from build123d import *

# Parameters (mm, degrees)
F0_R     = 25.4
F1_DEPTH = 25.4
F2_T     = -2.54
F3_R     = 10.031251
F4_DEPTH = 25.401


with BuildPart() as f1:
    # F0 (on Front) → F1 (new body)
    with BuildSketch(Plane.XZ):
        Circle(F0_R)
    extrude(amount=F1_DEPTH)

    # F2
    f2_openings = [f1.faces().sort_by_distance(p)[0] for p in [
        (0, 0, 0),
    ]]
    offset(amount=F2_T, openings=f2_openings)

    # F3 (on Right) → F4 (cut, through all)
    with BuildSketch(Plane.YZ):
        with Locations((-12.55889, 0)):
            Circle(F3_R)
    extrude(amount=-F4_DEPTH, mode=Mode.SUBTRACT)


solid = f1.part
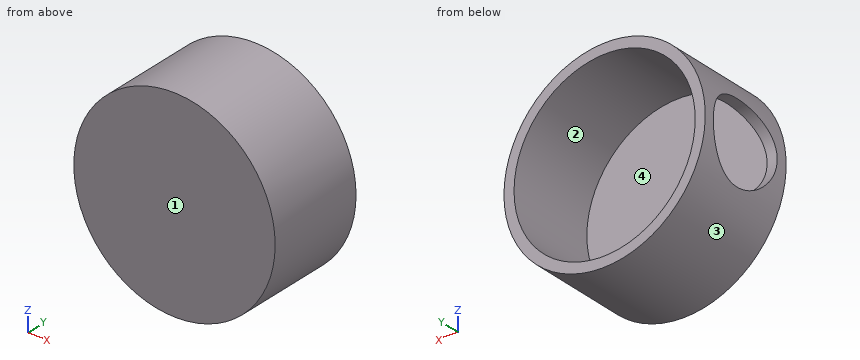
Source: CAD feature listing. Evaluate the final solid. Frame: model axes, mm. Face numbers are marked on the shaded views. Coordinates: 2 decimals unless noted, no trailing zeros. Loops run counter-clockwise (first coordinate to the right, second up) from the corner with the lowest first, then second, coordinate; pieces in that order, holes last. Notation, with made-up numbers: (23, 68.25) -> (59, 68.25) arc R13 ccw to (59, 76.25) -> close; hole circle Ø5 at (51, 62.5). An arc over 180 degrees is marked (long way). Answer in a Markdown table with one row per item. Add a question column.
Q1. Contact query for flat-ended pins moving along their axis: pin 1 Ø6 at (x, z) = (-7, 10.5) entering from +Y; pin 2 Ø10 at (x, y) = (-17.5, -4.5) entering from +Z; pin 3 Ø8 at (x, y) = (4, -20.5) entering from -Z. Output: stop coordinate, or through.
Q2. Section B-B on x = 0. Return the cut outline in (y, z), and give its area (3 significant figures).
Q3. Ray query, line 1 along Z through (x, y) = (0, -9.5); line 2 along Y through (x, z) = (1.5, 8.5); line 3 along X through (y, z) = (-7, 18). Return the intervals inside material, ascending.
Q4. Pull-direction query (X, two-part tool) for the marked faces 1, 2, 3 and 4; classes: pulls with the +X half, pulls with the -X half, needs draft (parallel to the pull), parting line crosses it, or undercut.
Q5. Section C-C on z = 19.5. Return the cut outline in (x, y), and give its area (3 significant figures).
Q6. Section A-A on z = 0. Return the cut outline in (x, y), and give its area (3 significant figures).
Q7. Section D-D on y = -15. Return the cut outline in (x, z).
Computed values:
| question | item | result |
|---|---|---|
| 1 | pin 1 | stops at y = -22.86 |
| 1 | pin 2 | stops at z = 22.11 |
| 1 | pin 3 | stops at z = -25.4 |
| 2 | outline | (-25.4, -25.4) -> (0, -25.4) -> (0, -22.86) -> (-22.86, -22.86) -> (-22.86, 22.86) -> (0, 22.86) -> (0, 25.4) -> (-25.4, 25.4) -> close |
| 2 | area | 245 mm^2 |
| 3 | line 1 | z = -25.4 to -22.86, 22.86 to 25.4 |
| 3 | line 2 | y = -25.4 to -22.86 |
| 3 | line 3 | x = -17.92 to -14.09, 14.09 to 17.92 |
| 4 | face 1 | needs draft |
| 4 | face 2 | undercut |
| 4 | face 3 | parting line crosses it |
| 4 | face 4 | undercut |
| 5 | outline | (-16.28, -25.4) -> (16.28, -25.4) -> (16.28, 0) -> (11.93, 0) -> (11.93, -22.86) -> (-11.93, -22.86) -> (-11.93, 0) -> (-16.28, 0) -> close |
| 5 | area | 281 mm^2 |
| 6 | outline | (-25.4, -25.4) -> (25.4, -25.4) -> (25.4, 0) -> (22.86, 0) -> (22.86, -22.86) -> (-22.86, -22.86) -> (-22.86, -22.59) -> (-25.4, -22.59) -> close; (-25.4, -2.53) -> (-22.86, -2.53) -> (-22.86, 0) -> (-25.4, 0) -> close |
| 6 | area | 194 mm^2 |
| 7 | outline | (-23.46, -9.73) arc R25.4 ccw (long way) to (-23.46, 9.73) -> (-20.69, 9.73) arc R22.86 cw (long way) to (-20.69, -9.73) -> close |
